from build123d import *

# Parameters (mm, degrees)
F0_W     = 76.2
F0_H     = 38.1
F1_DEPTH = 25.4
F2_W     = 25.4
F2_H     = 31.75
F3_DEPTH = 31.75
F4_R     = 6.35
F5_DEPTH = 25.4
F6_R     = 6.35
F7_DEPTH = 31.75


with BuildPart() as f1:
    # F0 (on Front) → F1 (new body)
    with BuildSketch(Plane.XZ):
        with Locations((-15.251094, 19.05)):
            Rectangle(F0_W, F0_H)
    extrude(amount=F1_DEPTH)

    # F2 (on face) → F3 (cut)
    with BuildSketch(Plane.XZ.offset(25.4)):
        with Locations((-40.651094, 22.225)):
            Rectangle(F2_W, F2_H)
        with Locations((10.148906, 22.225)):
            Rectangle(F2_W, F2_H)
    extrude(amount=-F3_DEPTH, mode=Mode.SUBTRACT)

    # F4 (on Top) → F5 (cut)
    with BuildSketch(Plane.XY):
        with Locations((10.148906, -12.7)):
            Circle(F4_R)
        with Locations((-40.651094, -12.7)):
            Circle(F4_R)
        with BuildLine():
            ThreePointArc((-40.651094, -25.4), (-49.63135, -21.680256), (-53.351094, -12.7))
            Line((-53.351094, -12.7), (-53.351094, -25.535107))
            Line((-53.351094, -25.535107), (-40.651094, -25.4))
        make_face()
        with BuildLine():
            ThreePointArc((-53.351094, -12.7), (-49.63135, -3.719744), (-40.651094, 0))
            Line((-40.651094, 0), (-53.351094, 0))
            Line((-53.351094, 0), (-53.351094, -12.7))
        make_face()
        with BuildLine():
            Line((22.848906, -25.4), (22.848906, -12.7))
            ThreePointArc((22.848906, -12.7), (19.129162, -21.680256), (10.148906, -25.4))
            Line((10.148906, -25.4), (22.848906, -25.4))
        make_face()
        with BuildLine():
            ThreePointArc((10.148906, 0), (19.129162, -3.719744), (22.848906, -12.7))
            Line((22.848906, -12.7), (22.848906, 0))
            Line((22.848906, 0), (10.148906, 0))
        make_face()
    extrude(amount=F5_DEPTH, mode=Mode.SUBTRACT)

    # F6 (on face) → F7 (cut)
    with BuildSketch(Plane.YZ.offset(-2.551094)):
        with Locations((-12.7, 25.4)):
            Circle(F6_R)
        with BuildLine():
            Line((0, 38.1), (-12.7, 38.1))
            ThreePointArc((-12.7, 38.1), (-3.719744, 34.380256), (0, 25.4))
            Line((0, 25.4), (0, 38.1))
        make_face()
        with BuildLine():
            ThreePointArc((-25.4, 25.4), (-21.680256, 34.380256), (-12.7, 38.1))
            Line((-12.7, 38.1), (-25.4, 38.1))
            Line((-25.4, 38.1), (-25.4, 25.4))
        make_face()
    extrude(amount=-F7_DEPTH, mode=Mode.SUBTRACT)


solid = f1.part
Model file for the job. Use its own axes, mm. A direction names the side the tool comes from. Give positions to 0.01 mm unless a question says otherwise; leave off trailing zeros. Order: outer loops, then holes, each group sorted by start corner. A loop starts at its lowest first (then second) coordinate and runs counter-clockwise, first axis right, second up. Notation, with made-up numbers: (85.25, 83.5) - (130.25, 83.5) arc R18 cw to (130.25, 97.5) - close; hole circle Ø5 at (11, -14.75). An arc over 180 degrees is marked (long way). One line per item, written item: value.
Item 1: Tool access for faces 4 (the flat face through (4, -16, 6.35)), 5 (the flat face through (-16, -13, 0)), 6 (the flat face through (-27.951, -13, 18)): list every direction of +Z, -Z, +X, -X, +Y, -Y with a clear straight run to the whole face (end or side of a thin tool).
Response values:
face 4: +Z, +X, +Y, -Y
face 5: -Z, +X, -X, +Y, -Y
face 6: +Z, -X, +Y, -Y
Item 2: Slice it at C-C (x = -23). List the corners of the cut face in (y, z).
Response values:
outline: (-25.4, 0) - (0, 0) - (0, 25.4) arc R12.7 ccw to (-25.4, 25.4) - close; hole circle Ø12.7 at (-12.7, 25.4)
Item 3: Wall check: line 1 (X direction, y = -10.25, z = 3.5); line 2 (X direction, y = -8.75, z = 5); line 3 (Z direction, x = -18.5, y = -12.7). Give the ranges that are in metal, low to high.
Response values:
line 1: -53.11 to -46.51, -34.79 to 4.29, 16.01 to 22.61
line 2: -52.72 to -45.62, -35.68 to 5.18, 15.12 to 22.22
line 3: 0 to 19.05, 31.75 to 38.1
Item 4: Slice it at B-B (y = -11.75). List the corners of the cut face in (x, z), then the cut area to 3 significant figures.
Response values:
outline: (-53.32, 0) - (-46.93, 0) - (-46.93, 6.35) - (-53.32, 6.35) - close; (-34.37, 0) - (3.87, 0) - (3.87, 6.35) - (-2.55, 6.35) - (-2.55, 19.12) - (-27.95, 19.12) - (-27.95, 6.35) - (-34.37, 6.35) - close; (-27.95, 31.68) - (-2.55, 31.68) - (-2.55, 38.06) - (-27.95, 38.06) - close; (16.43, 0) - (22.81, 0) - (22.81, 6.35) - (16.43, 6.35) - close
area: 811 mm2
Item 5: Slice it at D-D (z = 30.5). List the corners of the cut face in (x, y), then the cut area to 3 significant figures.
Response values:
outline: (-27.95, -24.33) - (-2.55, -24.33) - (-2.55, -16.48) - (-27.95, -16.48) - close; (-27.95, -8.92) - (-2.55, -8.92) - (-2.55, -1.07) - (-27.95, -1.07) - close
area: 399 mm2
Item 6: Slice it at A-A (z = 2.5). List the corners of the cut face in (x, y), then the cut area to 3 significant figures.
Response values:
outline: (-40.65, -25.4) - (10.15, -25.4) arc R12.7 ccw to (10.15, 0) - (-40.65, 0) arc R12.7 ccw to start; hole circle Ø12.7 at (-40.65, -12.7); hole circle Ø12.7 at (10.15, -12.7)
area: 1,540 mm2
Item 7: Two-plate mould, pull along Y, no slides. Class faces 1 (the cylindrical face through (13.079, -18.334, 3.131)), 2 (the flat face through (-38, -19, 6.35)), 3 (the flat face through (-16, 0, 10)): released by +Y, released by -Y, zero draft, split by the parting line, or undercut.
Response values:
face 1: undercut
face 2: zero draft
face 3: released by +Y
Item 8: Pin check, flat tips, straight feed: pin 1 Ø7.5 at (x, y) = (5.5, -10.5) entering from +Z; pin 2 Ø7.5 at (y, z) = (-18, 25.5) entering from -X; pin 3 Ø4 at (y, z) = (-15.5, 30) entering from +X. Stop position of each tip, or through.
Response values:
pin 1: z = 6.35
pin 2: x = -27.95
pin 3: x = -2.55
